Geometry check sheet. Reference: the model listing, model coordinates, mm. Face numbers are marked on the shaded views. A direction names the side the tool comes from. Round coordinates to 2 decimals unless told otherwise and drop trailing zeros. Write each loop counter-clockwise with the first axis right and the second up, starting at its lowest first coordinate (ties: lowest second). Pieces come first, ordered by that corner, then holes. Notation, with made-up numbers: M 59.5,2 L 105.5,2 A25 ccw 105.5,26 Z; hole C 46,-11.75 d3. An arc over 180 degrees is marked long. Use a Markdown table: item, result.
```python
from build123d import *
from OCP.BRepFilletAPI import BRepFilletAPI_MakeChamfer

# Parameters (mm, degrees)
BOSS_EXTRUDE1_DEPTH                    = 38.1
F_3_8_0_375_DIAMETER_HOLE1_D           = 9.525
F_3_8_0_375_DIAMETER_HOLE1_CSINK_D     = 10.795
F_3_8_0_375_DIAMETER_HOLE1_CSINK_ANGLE = 90
CHAMFER1_SIZE                          = 10.16
CHAMFER1_SIZE2                         = 5.865878735
FILLET1_R                              = 2.54
FILLET2_R                              = 6.35
CHAMFER2_SIZE                          = 0.254
CHAMFER2_SIZE2                         = 0.299341871
CHAMFER2_SIZE2_2                       = 0.693940905


with BuildPart() as part:
    # Sketch1 → Boss-Extrude1 (new body)
    with BuildSketch(Plane.XY):
        Polygon((0, 0), (30.988, 0), (30.988, -12.7), (-4.572, -12.7), (-4.572, -7.112), (-45.212, -7.112), (-45.212, 0), (-15.875, 0), (-9.525, 44.45), (0, 44.45), align=None)
    extrude(amount=BOSS_EXTRUDE1_DEPTH)

    # 3/8 (0.375) Diameter Hole1 (through all)
    with Locations(Plane(origin=(0, 0, 0), x_dir=(1, 0, 0), z_dir=(0, 1, 0))):
        with Locations((-30.5435, -19.05)):
            CounterSinkHole(F_3_8_0_375_DIAMETER_HOLE1_D / 2, F_3_8_0_375_DIAMETER_HOLE1_CSINK_D / 2, counter_sink_angle=F_3_8_0_375_DIAMETER_HOLE1_CSINK_ANGLE)

    # Chamfer1
    chamfer1_edges = [part.edges().sort_by_distance(p)[0] for p in [
        (30.988, -12.7, 19.05),
    ]]
    chamfer1_side = [part.faces().sort_by_distance(p)[0] for p in [
        (13.208, -12.7, 19.05),
    ]]
    chamfer(chamfer1_edges, length=CHAMFER1_SIZE, length2=CHAMFER1_SIZE2, reference=chamfer1_side[0])

    # Fillet1
    fillet1_edges = [part.edges().sort_by_distance(p)[0] for p in [
        (-15.875, 0, 19.05),
    ]]
    fillet(fillet1_edges, radius=FILLET1_R)

    # Fillet2
    fillet2_edges = [part.edges().sort_by_distance(p)[0] for p in [
        (0, 0, 19.05),
    ]]
    fillet(fillet2_edges, radius=FILLET2_R)

    # Chamfer2: one chamfer whose edges measure the first distance from different faces: ONE call of the kernel's chamfer builder (chamfer() names one face for all edges)
    chamfer2_edges_1 = [part.edges().sort_by_distance(p)[0] for p in [
        (30.988, 0, 19.05),
        (0, 44.45, 19.05),
    ]]
    chamfer2_edges_2 = [part.edges().sort_by_distance(p)[0] for p in [
        (-9.525, 44.45, 19.05),
    ]]
    chamfer2_side_2 = [part.faces().sort_by_distance(p)[0] for p in [
        (-4.7625, 44.45, 19.05),
    ]]
    chamfer2_edges_3 = [part.edges().sort_by_distance(p)[0] for p in [
        (30.988, -6.834121265, 19.05),
    ]]
    chamfer2_side_3 = [part.faces().sort_by_distance(p)[0] for p in [
        (25.908, -9.767060633, 19.05),
    ]]
    chamfer2 = BRepFilletAPI_MakeChamfer(part.part.solid().wrapped)
    for e in chamfer2_edges_1:
        chamfer2.Add(CHAMFER2_SIZE, e.wrapped)
    for e in chamfer2_edges_2:
        chamfer2.Add(CHAMFER2_SIZE, CHAMFER2_SIZE2, e.wrapped, chamfer2_side_2[0].wrapped)  # the first distance lies on this face
    for e in chamfer2_edges_3:
        chamfer2.Add(CHAMFER2_SIZE, CHAMFER2_SIZE2_2, e.wrapped, chamfer2_side_3[0].wrapped)  # the first distance lies on this face
    add(Compound.cast(chamfer2.Shape()), mode=Mode.REPLACE)


solid = part.part
```
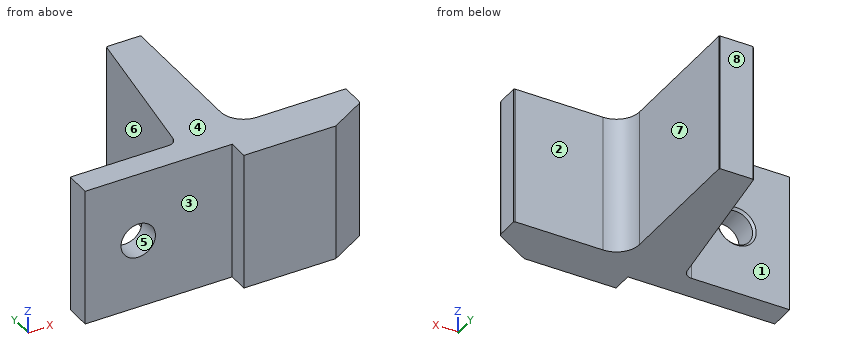
Item 1: Mould release check, pull along X, two halves, no side actions. Record for the marked faces 5, 6, 7 and 8: +X half, -X half, draft (parallel to the pull), parting line (faces both ways), or undercut.
Outcome:
| item | result |
|---|---|
| face 5 | undercut |
| face 6 | -X half |
| face 7 | +X half |
| face 8 | draft |
Item 2: Cross-section at A-A, the plane z = 19.05. Record the cut outline in (x, y) (3 decimals), and give its area (3 significant figures).
Outcome:
| item | result |
|---|---|
| outline | M -45.212,-7.112 L -35.306,-7.112 L -35.306,-0.635 L -35.941,0 L -45.212,0 Z; M -25.781,-7.112 L -4.572,-7.112 L -4.572,-12.7 L 20.828,-12.7 L 30.768,-6.961 L 30.988,-6.14 L 30.988,-0.254 L 30.734,0 L 6.35,0 A6.35 cw 0,6.35 L 0,44.196 L -0.254,44.45 L -9.271,44.45 L -9.567,44.154 L -15.563,2.181 A2.54 cw -18.078,0 L -25.146,0 L -25.781,-0.635 Z |
| area | 1,220 mm2 |
Item 3: Cross-section at C-C, the plane z = 28.5. Record the cut outline in (x, y), and give its area (3 significant figures).
Outcome:
| item | result |
|---|---|
| outline | M -45.21,-7.11 L -4.57,-7.11 L -4.57,-12.7 L 20.83,-12.7 L 30.77,-6.96 L 30.99,-6.14 L 30.99,-0.25 L 30.73,0 L 6.35,0 A6.35 cw 0,6.35 L 0,44.2 L -0.25,44.45 L -9.27,44.45 L -9.57,44.15 L -15.56,2.18 A2.54 cw -18.08,0 L -45.21,0 Z |
| area | 1,280 mm2 |
Item 4: Cross-section at D-D, the plane x = 8. Record the cut outline in (y, z), and give its area (3 significant figures).
Outcome:
| item | result |
|---|---|
| outline | M -12.7,0 L 0,0 L 0,38.1 L -12.7,38.1 Z |
| area | 484 mm2 |
Item 5: Go/stop test with flat-tipped pins: pin 1 (2 mm diameter, centred on x = 5, z = 19.5, fed in from +Y); pin 2 (4 mm diameter, centred on y = 26, z = 6.5, fed in from +X); pin 3 (11 mm diameter, centred on x = -30.54, z = 19.05, fed in from -Y). Record where each tip stops, or that it passes through.
Outcome:
| item | result |
|---|---|
| pin 1 | stops at y = 0.45 |
| pin 2 | stops at x = 0 |
| pin 3 | stops at y = -7.11 |
Item 6: Access from +Z, -Z, +X, -X, +Y, -Y to the whole of each face (thin tool, end or side, straight path). Record for the marked faces 1, 2, 3 and 4.
Outcome:
| item | result |
|---|---|
| face 1 | +Z, -Z, -X, +Y |
| face 2 | +Z, -Z, +X, +Y |
| face 3 | +Z, -Z, -X, -Y |
| face 4 | +Z, +X, -X, +Y, -Y |
Item 7: Material ranges on line 1 along X through (y, z) = (-3.25, 19.05); line 2 along Y through (x, z) = (-20, 32); line 3 along Y through (x, z) = (13.5, 10), recorded low to high. Write a range as from..to.
Outcome:
| item | result |
|---|---|
| line 1 | x = -45.21..-35.31, -25.78..30.99 |
| line 2 | y = -7.11..0 |
| line 3 | y = -12.7..0 |
